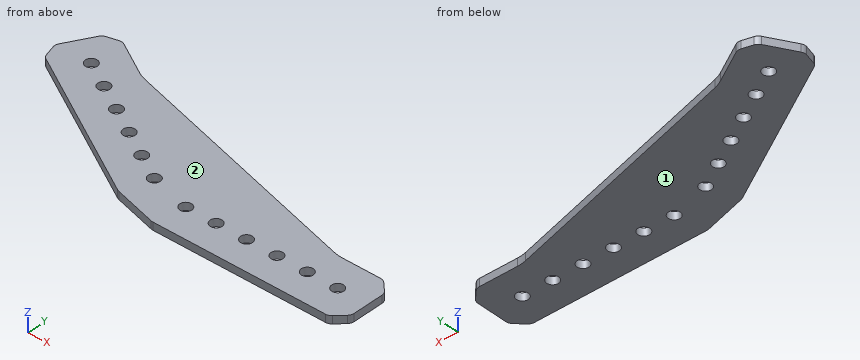
```python
from build123d import *

# Parameters (mm, degrees)
SKETCH1_R           = 2.4892
BOSS_EXTRUDE1_DEPTH = 3.175


with BuildPart() as part:
    # Sketch1 → Boss-Extrude1 (new body)
    with BuildSketch(Plane(origin=(0, 0, 0), x_dir=(-1, 0, 0), z_dir=(0, 0, -1))):
        with BuildLine():
            Line((-82.657359313, 0), (-10.394957493, 0))
            ThreePointArc((-10.394957493, 0), (-10.003378916, 0.025665416), (-9.618500357, 0.102222521))
            Line((-9.618500357, 0.102222521), (8.278754395, 4.897777479))
            ThreePointArc((8.278754395, 4.897777479), (8.650347557, 5.02391636), (9.00229726, 5.197478746))
            Line((9.00229726, 5.197478746), (71.583372975, 41.328679656))
            ThreePointArc((71.583372975, 41.328679656), (72.463432996, 42.100471581), (72.981150454, 43.150298732))
            Line((72.981150454, 43.150298732), (74.16803932, 47.579828286))
            ThreePointArc((74.16803932, 47.579828286), (74.244596426, 48.747863998), (73.868338053, 49.856285422))
            Line((73.868338053, 49.856285422), (67.41097874, 61.040759834))
            ThreePointArc((67.41097874, 61.040759834), (66.639186816, 61.920819855), (65.589359664, 62.438537313))
            Line((65.589359664, 62.438537313), (61.15983011, 63.62542618))
            ThreePointArc((61.15983011, 63.62542618), (59.991794398, 63.701983285), (58.883372975, 63.325724913))
            Line((58.883372975, 63.325724913), (45.095284847, 55.365168521))
            ThreePointArc((45.095284847, 55.365168521), (43.335536333, 54.49735659), (41.477570524, 53.866662183))
            Line((41.477570524, 53.866662183), (-62.853960852, 25.911112606))
            ThreePointArc((-62.853960852, 25.911112606), (-64.778353646, 25.528327079), (-66.736246529, 25.4))
            Line((-66.736246529, 25.4), (-82.657359313, 25.4))
            ThreePointArc((-82.657359313, 25.4), (-83.80540961, 25.171638598), (-84.778679656, 24.521320344))
            Line((-84.778679656, 24.521320344), (-88.021320344, 21.278679656))
            ThreePointArc((-88.021320344, 21.278679656), (-88.671638598, 20.30540961), (-88.9, 19.157359313))
            Line((-88.9, 19.157359313), (-88.9, 6.242640687))
            ThreePointArc((-88.9, 6.242640687), (-88.671638598, 5.09459039), (-88.021320344, 4.121320344))
            Line((-88.021320344, 4.121320344), (-84.778679656, 0.878679656))
            ThreePointArc((-84.778679656, 0.878679656), (-83.80540961, 0.228361402), (-82.657359313, 0))
        make_face()
        with Locations((-12.7, 12.7)):
            Circle(SKETCH1_R, mode=Mode.SUBTRACT)
        with Locations((4.648522628, 17.348522628)):
            Circle(SKETCH1_R, mode=Mode.SUBTRACT)
        with Locations((-63.5, 12.7)):
            Circle(SKETCH1_R, mode=Mode.SUBTRACT)
        with Locations((-38.1, 12.7)):
            Circle(SKETCH1_R, mode=Mode.SUBTRACT)
        with Locations((26.645567884, 30.048522628)):
            Circle(SKETCH1_R, mode=Mode.SUBTRACT)
        with Locations((48.64261314, 42.748522628)):
            Circle(SKETCH1_R, mode=Mode.SUBTRACT)
        with Locations((-76.2, 12.7)):
            Circle(SKETCH1_R, mode=Mode.SUBTRACT)
        with Locations((-50.8, 12.7)):
            Circle(SKETCH1_R, mode=Mode.SUBTRACT)
        with Locations((-25.4, 12.7)):
            Circle(SKETCH1_R, mode=Mode.SUBTRACT)
        with Locations((15.647045256, 23.698522628)):
            Circle(SKETCH1_R, mode=Mode.SUBTRACT)
        with Locations((37.644090512, 36.398522628)):
            Circle(SKETCH1_R, mode=Mode.SUBTRACT)
        with Locations((59.641135768, 49.098522628)):
            Circle(SKETCH1_R, mode=Mode.SUBTRACT)
    extrude(amount=-BOSS_EXTRUDE1_DEPTH)


solid = part.part
```
For this review, take the finished solid that the model builds, in its own axes (mm). Face numbers are marked on the shaded views. Round coordinates to 2 decimals unless told otherwise and drop trailing zeros. Write each loop counter-clockwise with the first axis right and the second up, starting at its lowest first coordinate (ties: lowest second). Pieces come first, ordered by that corner, then holes.
1) Take a section at A-A on x = 76.2. Give the boundary of the cut face in (y, z) (3 decimals), then the cut area to 3 significant figures.
Answer below:
outline: (0, 0) - (10.211, 0) - (10.211, 3.175) - (0, 3.175) - close; (15.189, 0) - (25.4, 0) - (25.4, 3.175) - (15.189, 3.175) - close
area: 64.8 mm2
2) Take a section at D-D on z = 0.75. State how many separate pieces and enclosed holes the cut face has, then the cut area to 3 significant figures.
Answer below:
separate pieces: 1
enclosed holes: 12
area: 4,870 mm2
3) Take a section at C-C on x = 12.7. Give the boundary of the cut face in (y, z) (3 decimals), then the cut area to 3 significant figures.
Answer below:
outline: (0, 0) - (10.211, 0) - (10.211, 3.175) - (0, 3.175) - close; (15.189, 0) - (39.35, 0) - (39.35, 3.175) - (15.189, 3.175) - close
area: 109 mm2
4) For line 1 along Y through (x, z) = (63.5, 0.45); line 2 along Y through (x, z) = (40, 1.55); line 3 along X through (y, z) = (7, 1.45), list the stretches that pass through material, from the lowest coordinate up.
Answer below:
line 1: y = 0 to 10.21, 15.19 to 25.75
line 2: y = 0 to 11.09, 14.31 to 32.03
line 3: x = -12.12 to 88.9
5) Take a section at B-B on y = 12.7. Give the boundary of the cut face in (x, z) (3 decimals).
Answer below:
outline: (-21.997, 0) - (10.211, 0) - (10.211, 3.175) - (-21.997, 3.175) - close; (15.189, 0) - (22.911, 0) - (22.911, 3.175) - (15.189, 3.175) - close; (27.889, 0) - (35.611, 0) - (35.611, 3.175) - (27.889, 3.175) - close; (40.589, 0) - (48.311, 0) - (48.311, 3.175) - (40.589, 3.175) - close; (53.289, 0) - (61.011, 0) - (61.011, 3.175) - (53.289, 3.175) - close; (65.989, 0) - (73.711, 0) - (73.711, 3.175) - (65.989, 3.175) - close; (78.689, 0) - (88.9, 0) - (88.9, 3.175) - (78.689, 3.175) - close
6) Insertion check: pin 1 Ø6.5 at (x, y) = (-15.65, 23.7) entering from -Z; pin 2 Ø1.5 at (x, z) = (-14, 1) entering from -Y. Each pin has a flat end and moves straight along its axis. Give the tip position at first contact, or say it passes through.
Answer below:
pin 1: stops at z = 0
pin 2: stops at y = 7.65
7) Mouldability with a two-part tool opening along Z and no side actions: class the marked faces 1 and 2 as +Z half, -Z half, draft (parallel to the pull), parting line (faces both ways), or undercut.
Answer below:
face 1: -Z half
face 2: +Z half
